Check sheet for the modelled part. Datum: model origin and axes. Units: mm. A direction names the side the tool comes from. Round coordinates to 2 decimals unless told otherwise and drop trailing zeros. Loops run counter-clockwise (first coordinate to the right, second up) from the corner with the lowest first, then second, coordinate; pieces in that order, holes last. Notation, with made-up numbers: M 83,73 L 134,73 A25 ccw 134,98 Z; hole C 76.5,-28.5 d11. An arc over 180 degrees is marked long. One line per question, with ' | ' between items. Start each with the question number.
(1) Section check B-B (z = 26). Record the boundary of the cut face in (x, y).
(2) Go/stop test with flat-tipped pins: P1, Ø12, axis at y = 20, z = 13, coming from the -X side; P2, Ø9, axis at y = 6, z = 24.5, coming from the +X side. Record where each tip stops, or that it passes through.
(3) Draft check along X on faces 3 (the face through (0, 3, 0)), 4 (the face through (0.66, 29.993, 1.942)), 5 (the face through (0, 15, 35)). Enter one of: +X half, -X half, draft (parallel to the pull), parting line (faces both ways), or undercut.
(4) Section check D-D (y = -2). Record the boundary of the cut face in (x, z).
(5) Section check C-C (y = 17). Record the boundary of the cut face in (x, z), and give its area (3 significant figures).
(6) Section check A-A (x = 0). Record the boundary of the cut face in (y, z), and give its area (3 significant figures).
(7) Tool access check on faces 1 (the face through (-25.07, -12.32, 19.72)), 2 (the face through (24, 9, 20)). Record the directions out of +Z, -Z, +X, -X, +Y, -Y that give a thin tool (end or side, any length) a straight path to the whole face; none if there is none.
(8) Thickness scan on probe 1 along Z at (x, y) = (8, 1); probe 2 along Y at (x, z) = (-14.5, 15.5); probe 3 along X at (y, z) = (2, 33.5). Record the ranges inside material, lowest first. Write a range as [from, to].
```python
from build123d import *

# Parameters (mm, degrees)
PAD_DEPTH    = 40
SKETCH001_W  = 48
SKETCH001_H  = 30
POCKET_DEPTH = 30


with BuildPart() as part:
    # Sketch → Pad (new body)
    with BuildSketch(Plane.XY):
        with BuildLine():
            ThreePointArc((30, 0), (0, 30), (-30, 0))
            Line((-30, 0), (-20, -25))
            Line((-20, -25), (20, -25))
            Line((20, -25), (30, 0))
        make_face()
    extrude(amount=PAD_DEPTH)

    # Sketch001 → Pocket (cut)
    with BuildSketch(Plane.XZ):
        with Locations((0, 20)):
            Rectangle(SKETCH001_W, SKETCH001_H)
    extrude(amount=-POCKET_DEPTH, mode=Mode.SUBTRACT)


solid = part.part
```
The answers:
1) outline: M -30,0 L -20,-25 L 20,-25 L 30,0 A30 ccw 24,18 L 24,0 L -24,0 L -24,18 A30 ccw Z
2) P1: x = -26.53 | P2: x = 29.96
3) face 3: draft | face 4: parting line | face 5: undercut
4) outline: M -29.2,0 L 29.2,0 L 29.2,40 L -29.2,40 Z
5) outline: M -24.72,0 L 24.72,0 L 24.72,40 L -24.72,40 Z; hole M -24,5 L 24,5 L 24,35 L -24,35 Z | area: 537 mm²
6) outline: M -25,0 L 30,0 L 30,5 L 0,5 L 0,35 L 30,35 L 30,40 L -25,40 Z | area: 1,300 mm²
7) face 1: +Z, -Z, -X, -Y | face 2: +Y
8) probe 1: [0, 5], [35, 40] | probe 2: [-25, 0] | probe 3: [-29.93, -24], [24, 29.93]
